from build123d import *

# Parameters (mm, degrees)
SKETCH1_W               = 150
SKETCH1_H               = 20
BOSS_EXTRUDE1_DEPTH     = 10
BOSS_EXTRUDE2_DEPTH     = 10
CUT_EXTRUDE1_DEPTH      = 80.930394481
CUT_EXTRUDE1_DEPTH_BACK = 80.930394481
SKETCH3_R               = 2
SKETCH4_W               = 7
SKETCH4_H               = 2.9
CUT_EXTRUDE2_DEPTH      = 13.8
CUT_EXTRUDE3_DEPTH      = 82.785499704
CUT_EXTRUDE3_DEPTH_BACK = 82.785499704
SKETCH4_3_R             = 2


with BuildPart() as part:
    # Sketch1 → Boss-Extrude1 (new body)
    with BuildSketch(Plane(origin=(0, 0, 0), x_dir=(1, 0, 0), z_dir=(0, 1, 0))):
        Rectangle(SKETCH1_W, SKETCH1_H)
    extrude(amount=BOSS_EXTRUDE1_DEPTH)

    # Sketch2 → Boss-Extrude2 (add, symmetric)
    with BuildSketch(Plane.XY):
        Polygon((-75, 10), (75, 10), (75, 25.76563529), align=None)
    extrude(amount=BOSS_EXTRUDE2_DEPTH, both=True)

    # Sketch3 → Cut-Extrude1 (cut, two sides: drawn at the far end of the back side and taken through both)
    with BuildSketch(Plane.XZ.offset(-CUT_EXTRUDE1_DEPTH_BACK)):
        with Locations(Location((15, 0, 0), (0, 0, 270))):
            Circle(SKETCH3_R)
    extrude(amount=CUT_EXTRUDE1_DEPTH + CUT_EXTRUDE1_DEPTH_BACK, mode=Mode.SUBTRACT)

    # Sketch4 → Cut-Extrude2 (cut)
    with BuildSketch(Plane.XY.offset(10)):
        with Locations((15, 6.45)):
            Rectangle(SKETCH4_W, SKETCH4_H)
    extrude(amount=-CUT_EXTRUDE2_DEPTH, mode=Mode.SUBTRACT)

    # Sketch4_3 → Cut-Extrude3 (cut, two sides: drawn at the far end of the back side and taken through both)
    with BuildSketch(Plane.XY.offset(10).offset(-CUT_EXTRUDE3_DEPTH_BACK)):
        with Locations((-9.492687022, 11.857554637)):
            Circle(SKETCH4_3_R)
        with Locations((45.186458968, 17.604564461)):
            Circle(SKETCH4_3_R)
    extrude(amount=CUT_EXTRUDE3_DEPTH + CUT_EXTRUDE3_DEPTH_BACK, mode=Mode.SUBTRACT)


solid = part.part
Verification items for the finished model (mm, model axes). A direction names the side the tool comes from. Coordinates: 2 decimals unless noted, no trailing zeros. Loops run counter-clockwise (first coordinate to the right, second up) from the corner with the lowest first, then second, coordinate; pieces in that order, holes last. Notation, with made-up numbers: (19.5, 87.25) -> (39.5, 87.25) arc R22 ccw to (39.5, 111.25) -> close; hole circle Ø3 at (15, -32.5). An arc over 180 degrees is marked (long way). Answer as a JSON object with one key per item and string values. Group by question number.
Item 1: Mould release check, pull along Z, two halves, no side actions. Record for faces 1 (the cylindrical face through (17, 3, 0)), 2 (the flat face through (18.5, 6, 3)), 3 (the flat face through (15, 6, -3.8)): +Z half, -Z half, draft (parallel to the pull), parting line (faces both ways), or undercut.
Item 2: Scan lines: probe 1 along Z at (x, y) = (15, 12.5); probe 2 along X at (y, z) = (3.5, 0); probe 3 along Y at (x, z) = (16, 2). Record each from-to range of solid material in increasing order.
Item 3: Sectioned sample at A-A on z = 0. Record the boundary of the cut face in (x, y).
Item 4: Sectioned sample at B-B on y = 6.5. Record the boundary of the cut face in (x, z).
Item 5: Tool access check on faces 4 (the flat face through (-75, 5, 0)), 5 (the flat face through (15, 7.9, 3)). Record the directions out of +Z, -Z, +X, -X, +Y, -Y that give a thin tool (end or side, any length) a straight path to the whole face; none if there is none.
Item 6: Depth check by flat-ended pin: pin 1 (4.5 mm diameter, centred on x = 15, z = 0, fed in from +Y); pin 2 (12 mm diameter, centred on x = -21.5, z = 0.5, fed in from +Y); pin 3 (5 mm diameter, centred on x = -45, z = 1, fed in from -Y); pin 4 (7.5 mm diameter, centred on x = 16.5, z = 6, fed in from +Y). Enter the tip coordinate at first touch or a pass-through.
Item 7: Sectioned sample at D-D on z = -7.25. Record the boundary of the cut face in (x, y), plus the area to 3 significant figures.
Item 8: Sectioned sample at C-C on x = 15. Record the boundary of the cut face in (y, z), plus the area to 3 significant figures.
Evaluation:
{
 "1": {"face 1": "undercut", "face 2": "draft", "face 3": "+Z half"},
 "2": {"probe 1": "z = -10 to -2, 2 to 10", "probe 2": "x = -75 to 13, 17 to 75", "probe 3": "y = 0 to 5, 7.9 to 19.56"},
 "3": {"outline": "(-75, 0) -> (13, 0) -> (13, 5) -> (11.5, 5) -> (11.5, 7.9) -> (13, 7.9) -> (13, 19.25) -> (-75, 10) -> close; (17, 0) -> (75, 0) -> (75, 25.77) -> (17, 19.67) -> (17, 7.9) -> (18.5, 7.9) -> (18.5, 5) -> (17, 5) -> close; hole circle Ø4 at (-9.49, 11.86); hole circle Ø4 at (45.19, 17.6)"},
 "4": {"outline": "(-75, -10) -> (75, -10) -> (75, 10) -> (18.5, 10) -> (18.5, -3.8) -> (11.5, -3.8) -> (11.5, 10) -> (-75, 10) -> close"},
 "5": {"face 4": "+Z, -Z, -X, +Y, -Y", "face 5": "+Z"},
 "6": {"pin 1": "stops at y = 19.7", "pin 2": "stops at y = 16.25", "pin 3": "stops at y = 0", "pin 4": "stops at y = 20.01"},
 "7": {"outline": "(-75, 0) -> (75, 0) -> (75, 25.77) -> (-75, 10) -> close; hole circle Ø4 at (-9.49, 11.86); hole circle Ø4 at (45.19, 17.6)", "area": "2,660 mm²"},
 "8": {"outline": "(0, -10) -> (19.46, -10) -> (19.46, -2) -> (7.9, -2) -> (7.9, -3.8) -> (5, -3.8) -> (5, -2) -> (0, -2) -> close; (0, 2) -> (5, 2) -> (5, 10) -> (0, 10) -> close; (7.9, 2) -> (19.46, 2) -> (19.46, 10) -> (7.9, 10) -> close", "area": "283 mm²"}
}
